Geometry check sheet. Reference: drawing and pictorial views, mm from the part's lowest x, y, z. Round coordinates to 2 decimals unless told otherwise and drop trailing zeros. Write each loop counter-clockwise with the first axis right and the second up, starting at its lowest first coordinate (ties: lowest second). Pieces come first, ordered by that corner, then holes.
Item 1: Section check A-A, the plane y = 14.25. Record the cut outline in (x, z).
Item 2: Section check B-B, the plane x = 15.25. Record the cut outline in (y, z), plus the area to 3 significant figures.
Item 3: Release check for a two-part mould opening along Y. For the marked faces 1, 2 and 3 record: pulls with the +Y half, pulls with the -Y half, needs draft (parallel to the pull), parting line crosses it, or undercut.
Item 4: Section check C-C, the plane z = 116. Record the cut outline in (x, y).
Item 5: Material ranges on line 1 along X through (y, z) = (17.25, 65.5); line 2 along X through (y, z) = (18.75, 30); line 3 along Y through (x, z) = (8.75, 124.5), recorded low to high.
Item 6: Depth check by flat-ended pin: pin 1 (10 mm diameter, centred on x = 9, z = 43.5, fed in from -Y); pin 2 (9.5 mm diameter, centred on x = 13.5, y = 8.5, fed in from +Z). Enter the tip coordinate at first touch or a pass-through.
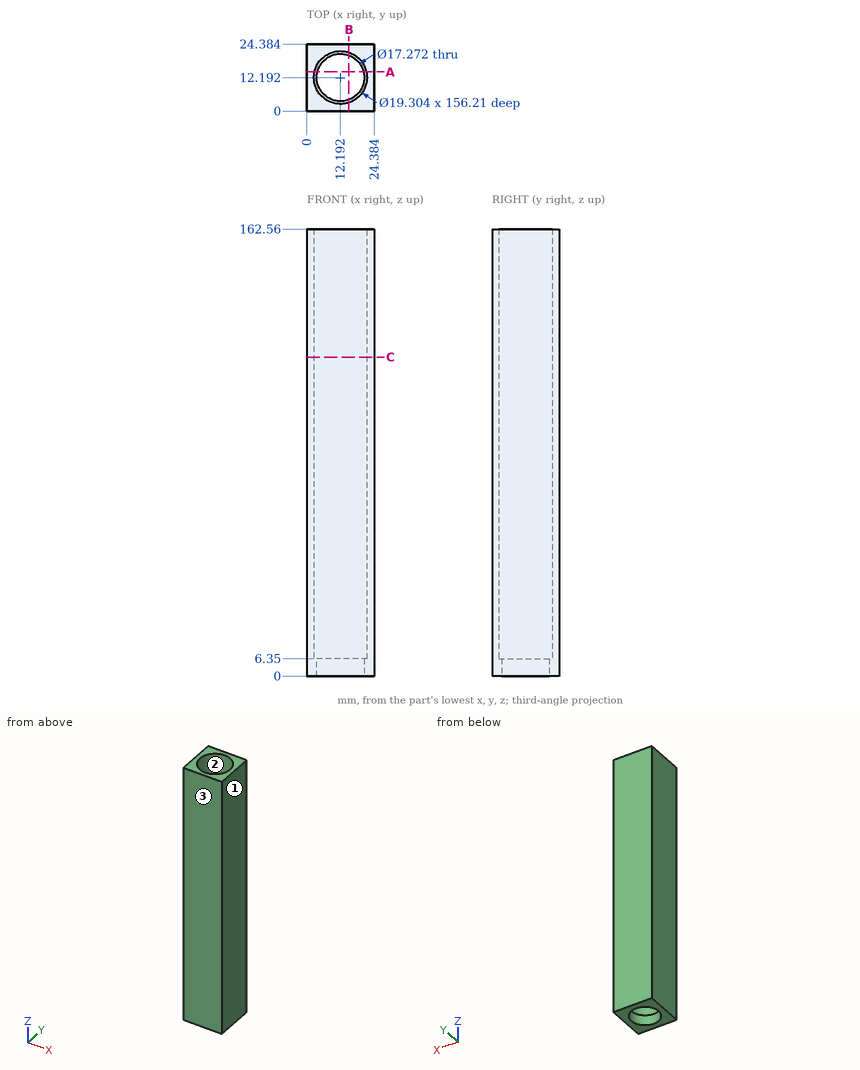
Values found:
1. outline: (0, 0) - (3.8, 0) - (3.8, 6.35) - (2.76, 6.35) - (2.76, 162.56) - (0, 162.56) - close; (20.58, 0) - (24.38, 0) - (24.38, 162.56) - (21.62, 162.56) - (21.62, 6.35) - (20.58, 6.35) - close
2. outline: (0, 0) - (4.12, 0) - (4.12, 6.35) - (3.04, 6.35) - (3.04, 162.56) - (0, 162.56) - close; (20.27, 0) - (24.38, 0) - (24.38, 162.56) - (21.35, 162.56) - (21.35, 6.35) - (20.27, 6.35) - close
2. area: 1,000 mm2
3. face 1: needs draft
3. face 2: undercut
3. face 3: pulls with the -Y half
4. outline: (0, 0) - (24.38, 0) - (24.38, 24.38) - (0, 24.38) - close; hole circle Ø19.3 at (12.19, 12.19)
5. line 1: x = 0 to 3.97, 20.41 to 24.38
5. line 2: x = 0 to 5.11, 19.27 to 24.38
5. line 3: y = 0 to 3.17, 21.21 to 24.38
6. pin 1: stops at y = 0
6. pin 2: stops at z = 6.35
